Geometry: final body of the model. Coordinates: model frame, mm. A direction names the side the tool comes from. Give positions to 0.01 mm unless a question says otherwise; leave off trailing zeros. Write each loop counter-clockwise with the first axis right and the second up, starting at its lowest first coordinate (ties: lowest second). Pieces come first, ordered by that corner, then holes. Notation, with made-up numbers: (-28, -1.5) -> (24, -1.5) arc R30 cw to (24, 35.5) -> close; hole circle Ø3 at (-9.75, -26). An arc over 180 degrees is marked (long way). Answer as a JSON object with one key per item and string values.
from build123d import *

# Parameters (mm, degrees)
SKETCH1_W               = 14.5
SKETCH1_H               = 8
BOSS_EXTRUDE1_DEPTH     = 23
CUT_EXTRUDE1_DEPTH      = 29.341665442
CUT_EXTRUDE1_DEPTH_BACK = 29.341665442
SKETCH2_W               = 2
SKETCH2_H               = 12.8


with BuildPart() as part:
    # Sketch1 → Boss-Extrude1 (new body)
    with BuildSketch(Plane.XY):
        with Locations((7.25, 4)):
            Rectangle(SKETCH1_W, SKETCH1_H)
    extrude(amount=BOSS_EXTRUDE1_DEPTH)

    # Sketch2 → Cut-Extrude1 (cut, two sides: drawn at the far end of the back side and taken through both)
    with BuildSketch(Plane.XZ.offset(-CUT_EXTRUDE1_DEPTH_BACK)):
        with Locations((7.25, 16.6)):
            Rectangle(SKETCH2_W, SKETCH2_H)
    extrude(amount=CUT_EXTRUDE1_DEPTH + CUT_EXTRUDE1_DEPTH_BACK, mode=Mode.SUBTRACT)


solid = part.part
Q1. Set-up query: faces 1 (the flat face through (8.25, 4, 17)), 2 (the flat face through (3, 4, 23)). Return all of +Z, -Z, +X, -X, +Y, -Y with unobstructed straight access to the full face (end or side cutting, diameter ignored); none if empty.
Values:
{"face 1": "+Z, +Y, -Y", "face 2": "+Z, +X, -X, +Y, -Y"}
Q2. Cut plane B-B (y = 5). Return the cut outline in (x, z).
Values:
{"outline": "(0, 0) -> (14.5, 0) -> (14.5, 23) -> (8.25, 23) -> (8.25, 10.2) -> (6.25, 10.2) -> (6.25, 23) -> (0, 23) -> close"}
Q3. Cut plane C-C (x = 7). Return the cut outline in (y, z), and give its area (3 significant figures).
Values:
{"outline": "(0, 0) -> (8, 0) -> (8, 10.2) -> (0, 10.2) -> close", "area": "81.6 mm²"}
Q4. Cut plane A-A (z = 21.25). Return the cut outline in (x, y).
Values:
{"outline": "(0, 0) -> (6.25, 0) -> (6.25, 8) -> (0, 8) -> close; (8.25, 0) -> (14.5, 0) -> (14.5, 8) -> (8.25, 8) -> close"}
Q5. Material intervals for L1, parallel to X at y = 5, z = 10.25; L2, parallel to Z at x = 7, y = 3.5, sorted ascending. Write a range as from..to.
Values:
{"L1": "0..6.25, 8.25..14.5", "L2": "0..10.2"}
Q6. Mould query, pull axis X, two halves, no side actions, for faces 3 (the flat face through (7, 4, 0)), 4 (the flat face through (14.5, 4, 11)), 5 (the flat face through (0, 4, 11)), 6 (the flat face through (6.25, 4, 17)). Classes: pulls with the +X half, pulls with the -X half, needs draft (parallel to the pull), parting line crosses it, or undercut.
Values:
{"face 3": "needs draft", "face 4": "pulls with the +X half", "face 5": "pulls with the -X half", "face 6": "undercut"}
